```python
from build123d import *

# Parameters (mm, degrees)
SALIENTE_EXTRUIR1_OUTLINE_W   = 123.605310211
SALIENTE_EXTRUIR1_OUTLINE_H   = 128.516462854
SALIENTE_EXTRUIR1_OUTLINE_R   = 2.5
SALIENTE_EXTRUIR1_OUTLINE_W_2 = 77.478408342
SALIENTE_EXTRUIR1_OUTLINE_H_2 = 109.077461589
SALIENTE_EXTRUIR1_DEPTH       = 8
REDONDEO1_R                   = 40
CROQUIS2_W                    = 8
CROQUIS2_H                    = 170
SALIENTE_EXTRUIR2_DEPTH       = 5
CROQUIS3_W                    = 8
CROQUIS3_H                    = 170
SALIENTE_EXTRUIR3_DEPTH       = 30
CROQUIS4_W                    = 8
CROQUIS4_H                    = 170
SALIENTE_EXTRUIR4_DEPTH       = 30
CROQUIS5_R                    = 3
CORTAR_EXTRUIR1_DEPTH         = 30


# Read off the part's stored shape, not the designer's step: Saliente-Extruir1
with BuildPart() as part:
    # Saliente-Extruir1 outline → Saliente-Extruir1 (new body)
    with BuildSketch(Plane(origin=(0, 0, -35.287768798), x_dir=(-1, 0, 0), z_dir=(0, 0, -1))):
        Polygon((-7.340270166, -457.935763063), (284.299805756, -457.935763063), (284.299805756, -113.999224426), (537.787991057, -113.999224426), (537.787991057, 56.000775574), (-51.831359741, 56.000775574), (-51.831359741, -113.999224426), (-7.340270166, -113.999224426), align=None)
        with Locations((116.749910344, -206.634344557)):
            Rectangle(SALIENTE_EXTRUIR1_OUTLINE_W, SALIENTE_EXTRUIR1_OUTLINE_H, mode=Mode.SUBTRACT)
        with Locations((54.137991057, -101.999224426)):
            Circle(SALIENTE_EXTRUIR1_OUTLINE_R, mode=Mode.SUBTRACT)
        with Locations((54.137991057, -81.499224426)):
            Circle(SALIENTE_EXTRUIR1_OUTLINE_R, mode=Mode.SUBTRACT)
        with Locations((-1.387076296, -11.960493631)):
            Rectangle(SALIENTE_EXTRUIR1_OUTLINE_W_2, SALIENTE_EXTRUIR1_OUTLINE_H_2, mode=Mode.SUBTRACT)
        with Locations((54.137991057, 23.500775574)):
            Circle(SALIENTE_EXTRUIR1_OUTLINE_R, mode=Mode.SUBTRACT)
        with Locations((54.137991057, 44.000775574)):
            Circle(SALIENTE_EXTRUIR1_OUTLINE_R, mode=Mode.SUBTRACT)
        with Locations((531.437991057, -101.999224426)):
            Circle(SALIENTE_EXTRUIR1_OUTLINE_R, mode=Mode.SUBTRACT)
        with Locations((531.437991057, -81.499224426)):
            Circle(SALIENTE_EXTRUIR1_OUTLINE_R, mode=Mode.SUBTRACT)
        with Locations((531.437991057, 23.500775574)):
            Circle(SALIENTE_EXTRUIR1_OUTLINE_R, mode=Mode.SUBTRACT)
        with Locations((531.437991057, 44.000775574)):
            Circle(SALIENTE_EXTRUIR1_OUTLINE_R, mode=Mode.SUBTRACT)
    extrude(amount=SALIENTE_EXTRUIR1_DEPTH)

    # Redondeo1
    redondeo1_edges = [part.edges().sort_by_distance(p)[0] for p in [
        (-54.947255239, -142.37611313, -39.287768798),
        (-54.947255239, -270.892575984, -39.287768798),
        (-178.55256545, -270.892575984, -39.287768798),
        (-178.55256545, -142.37611313, -39.287768798),
        (7.340270166, -113.999224426, -39.287768798),
        (-284.299805756, -113.999224426, -39.287768798),
    ]]
    fillet(redondeo1_edges, radius=REDONDEO1_R)

    # Croquis2 → Saliente-Extruir2 (add)
    with BuildSketch(Plane.ZY.offset(537.787991057)):
        with Locations((-39.287768798, -28.999224426)):
            Rectangle(CROQUIS2_W, CROQUIS2_H)
    extrude(amount=SALIENTE_EXTRUIR2_DEPTH)

    # Croquis3 → Saliente-Extruir3 (add)
    with BuildSketch(Plane.ZY.offset(542.787991057)):
        with Locations((-39.287768798, -28.999224426)):
            Rectangle(CROQUIS3_W, CROQUIS3_H)
    extrude(amount=SALIENTE_EXTRUIR3_DEPTH)

    # Croquis4 → Saliente-Extruir4 (add)
    with BuildSketch(Plane(origin=(51.831359741, 0, 0), x_dir=(0, 0, -1), z_dir=(1, 0, 0))):
        with Locations((39.287768798, -28.999224426)):
            Rectangle(CROQUIS4_W, CROQUIS4_H)
    extrude(amount=SALIENTE_EXTRUIR4_DEPTH)

    # Croquis5 → Cortar-Extruir1 (cut)
    with BuildSketch(Plane(origin=(0, 0, -43.287768798), x_dir=(-1, 0, 0), z_dir=(0, 0, -1))):
        with Locations((8.841068429, -446.316406302)):
            Circle(CROQUIS5_R)
        with Locations((8.841068429, -326.316406302)):
            Circle(CROQUIS5_R)
        with Locations((139.33299328, -326.316406302)):
            Circle(CROQUIS5_R)
        with Locations((269.824918132, -326.316406302)):
            Circle(CROQUIS5_R)
        with Locations((269.824918132, -446.316406302)):
            Circle(CROQUIS5_R)
    extrude(amount=-CORTAR_EXTRUIR1_DEPTH, mode=Mode.SUBTRACT)


solid = part.part
```
Check sheet for the modelled part. Datum: model origin and axes. Units: mm. A direction names the side the tool comes from. Coordinates: 2 decimals unless noted, no trailing zeros. Order: outer loops, then holes, each group sorted by start corner. A loop starts at its lowest first (then second) coordinate and runs counter-clockwise, first axis right, second up. Notation, with made-up numbers: M 55.5,-26 L 72.5,-26 A20 ccw 72.5,-2 Z; hole C 57.25,79.25 d7. An arc over 180 degrees is marked long. Write each question's results on one line, items separated by ' | '. Start each with the question number.
1. Cross-section at C-C on z = -41.25. State how many separate pieces and enclosed holes the cut face has, and give its area (3 significant figures).
2. Mould release check, pull along Y, two halves, no side actions. Record for faces 3 (the face through (-177, -147, -35.288)), 4 (the face through (-295.706, -126.028, -39.344)), 5 (the face through (-66.354, -154.405, -39.344)): +Y half, -Y half, draft (parallel to the pull), parting line (faces both ways), or undercut.
3. Cross-section at A-A on y = -14.5. Record the cut outline in (x, z), and give its area (3 significant figures).
4. Access from +Z, -Z, +X, -X, +Y, -Y to the whole of each face (thin tool, end or side, straight path). Record for faces 1 (the face through (-177, -147, -43.288)), 2 (the face through (-166.52, -259.49, -39.34)).
5. Cross-section at B-B on x = -502.5. Record the cut outline in (y, z).
6. Go/stop test with flat-tipped pins: P1, Ø3, axis at x = -54.14, y = 44, coming from the -Z side; P2, Ø4, axis at y = -169.5, z = -36.5, coming from the +X side; P3, Ø2.5, axis at x = 57, z = -40, coming from the -Y side; P4, Ø4, axis at y = -216, z = -39, coming from the -X side. Record where each tip stops, or that it passes through.
7. Cross-section at D-D on y = -246.5. Record the cut outline in (x, z), and give its area (3 significant figures).
8. Material ranges on probe 1 along X at (y, z) = (28, -38.5); probe 2 along X at (y, z) = (-188, -41); probe 3 along Y at (x, z) = (-131.5, -38.5), recorded low to high.
Checks:
1) separate pieces: 1 | enclosed holes: 15 | area: 189,000 mm²
2) face 3: draft | face 4: -Y half | face 5: undercut
3) outline: M -572.79,-43.29 L -37.35,-43.29 L -37.35,-35.29 L -572.79,-35.29 Z; M 40.13,-43.29 L 81.83,-43.29 L 81.83,-35.29 L 40.13,-35.29 Z | area: 4,620 mm²
4) face 1: -Z, +X, -X, +Y, -Y | face 2: +Z, -Z
5) outline: M -114,-43.29 L 56,-43.29 L 56,-35.29 L -114,-35.29 Z
6) P1: passes through | P2: stops at x = 7.34 | P3: stops at y = -114 | P4: stops at x = -284.3
7) outline: M -284.3,-43.29 L -175.38,-43.29 L -175.38,-35.29 L -284.3,-35.29 Z; M -58.12,-43.29 L 7.34,-43.29 L 7.34,-35.29 L -58.12,-35.29 Z | area: 1,400 mm²
8) probe 1: x = -572.79 to -37.35, 40.13 to 81.83 | probe 2: x = -284.3 to -178.55, -54.95 to 7.34 | probe 3: y = -457.94 to -270.89, -142.38 to 56
